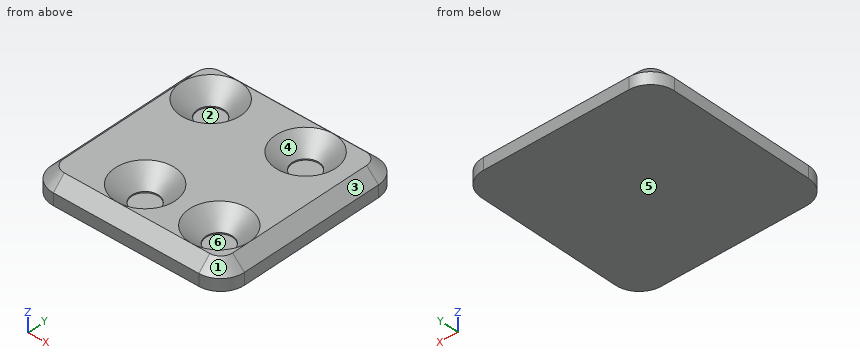
from build123d import *

# Parameters (mm, degrees)
SKETCH1_W           = 32.526911934
SKETCH1_H           = 32.526911934
BOSS_EXTRUDE1_DEPTH = 4
FILLET1_R           = 4
CHAMFER1_SIZE       = 2
SKETCH2_R           = 2.25
CUT_EXTRUDE1_DEPTH  = 3
CHAMFER2_SIZE       = 2.8


with BuildPart() as part:
    # Sketch1 → Boss-Extrude1 (new body)
    with BuildSketch(Plane.XY):
        Rectangle(SKETCH1_W, SKETCH1_H)
    extrude(amount=BOSS_EXTRUDE1_DEPTH)

    # Fillet1
    fillet1_edges = [part.edges().sort_by_distance(p)[0] for p in [
        (-16.263455967, 16.263455967, 2),
        (16.263455967, 16.263455967, 2),
        (16.263455967, -16.263455967, 2),
        (-16.263455967, -16.263455967, 2),
    ]]
    fillet(fillet1_edges, radius=FILLET1_R)

    # Chamfer1
    chamfer1_edges = [part.edges().sort_by_distance(p)[0] for p in [
        (0, -16.263455967, 4),
        (-16.263455967, 0, 4),
        (16.263455967, 0, 4),
        (0, 16.263455967, 4),
        (-15.091883092, 15.091883092, 4),
        (15.091883092, 15.091883092, 4),
        (15.091883092, -15.091883092, 4),
        (-15.091883092, -15.091883092, 4),
    ]]
    chamfer(chamfer1_edges, length=CHAMFER1_SIZE)

    # Sketch2 → Cut-Extrude1 (cut)
    with BuildSketch(Plane.XY.offset(4)):
        with Locations((-9.213455967, 9.213455967)):
            Circle(SKETCH2_R)
        with Locations((9.213455967, -9.213455967)):
            Circle(SKETCH2_R)
        with Locations((-3.286544033, -9.213455967)):
            Circle(SKETCH2_R)
        with Locations((6.786544033, 9.213455967)):
            Circle(SKETCH2_R)
    extrude(amount=-CUT_EXTRUDE1_DEPTH, mode=Mode.SUBTRACT)

    # Chamfer2
    chamfer2_edges = [part.edges().sort_by_distance(p)[0] for p in [
        (-11.463455967, 9.213455967, 4),
        (6.963455967, -9.213455967, 4),
        (-5.536544033, -9.213455967, 4),
        (4.536544033, 9.213455967, 4),
    ]]
    chamfer(chamfer2_edges, length=CHAMFER2_SIZE - 0.0001)  # a hair under: the kernel refuses the full size


solid = part.part
Work out the finished part from the listing and answer in its coordinate system (mm). Face numbers are marked on the shaded views. A direction names the side the tool comes from. Coordinates: 2 decimals unless noted, no trailing zeros. Order: outer loops, then holes, each group sorted by start corner. A loop starts at its lowest first (then second) coordinate and runs counter-clockwise, first axis right, second up. Notation, with made-up numbers: (50.5, 16.25) - (63.5, 16.25) arc R20 cw to (63.5, 27.25) - close; hole circle Ø5 at (-15, 4.5). An arc over 180 degrees is marked (long way). Put each result on its own line as item: value. Start each with the question number.
1) For the marked faces 5 and 6, determine the directions among +Z, -Z, +X, -X, +Y, -Y from which every point of the face is accessible in a straight line to the end or side of a thin tool.
2) Flat-ended cylindrical pins translate along their axes: pin 1 (5 mm diameter, centred on x = -9.21, y = 9.21, fed in from +Z) (3 decimals); pin 2 (5 mm diameter, centred on x = 9, y = -8.5, fed in from +Z); pin 3 (4 mm diameter, centred on x = 0, y = -12, fed in from +Z); pin 4 (2.5 mm diameter, centred on x = -3.29, y = -9.21, fed in from +Z). Find the tip coordinate at first contact, or state that the pin passes through.
3) For a pull along Y with two mould halves and no side action, classify the marked faces 1, 2, 3 and 4 as released by +Y, released by -Y, zero draft, split by the parting line, or undercut.
4) Find section B-B (y = 0). Give the vertices of the cut face in (x, z), plus the area to 3 significant figures.
5) Find the intervals of material crossed by line 1 (X direction, y = 11, z = 1.8); line 2 (X direction, y = 12, z = 3.75); line 3 (Y direction, x = -2, z = 2.25), in increasing order. Write a range as from..to.
6) Find section A-A (z = 3.25). Give the vertices of the cut face in (x, y).
Results list:
1. face 5: -Z, +X, -X, +Y, -Y
1. face 6: +Z
2. pin 1: stops at z = 1.455
2. pin 2: stops at z = 2.19
2. pin 3: stops at z = 4
2. pin 4: stops at z = 1
3. face 1: released by -Y
3. face 2: undercut
3. face 3: zero draft
3. face 4: undercut
4. outline: (-16.26, 0) - (16.26, 0) - (16.26, 2) - (14.26, 4) - (-14.26, 4) - (-16.26, 2) - close
4. area: 126 mm^2
5. line 1: x = -16.26..-11.43, -6.99..4.57, 9.01..16.26
5. line 2: x = -14.51..-13.12, -5.31..2.88, 10.69..14.51
5. line 3: y = -16.01..-12.25, -6.17..16.01
6. outline: (-15.01, -12.26) arc R2.75 ccw to (-12.26, -15.01) - (12.26, -15.01) arc R2.75 ccw to (15.01, -12.26) - (15.01, 12.26) arc R2.75 ccw to (12.26, 15.01) - (-12.26, 15.01) arc R2.75 ccw to (-15.01, 12.26) - close; hole circle Ø8.6 at (-9.21, 9.21); hole circle Ø8.6 at (-3.29, -9.21); hole circle Ø8.6 at (6.79, 9.21); hole circle Ø8.6 at (9.21, -9.21)
